from build123d import *

# Parameters (mm, degrees)
F0_R     = 30
F1_DEPTH = 5
F3_DEPTH = 5.001
F4_R     = 9.975
F5_DEPTH = 4.9


with BuildPart() as f1:
    # F0 (on Front) → F1 (new body)
    with BuildSketch(Plane.XZ):
        Circle(F0_R)
    extrude(amount=F1_DEPTH)

    # F2 (on face) → F3 (cut, through all)
    with BuildSketch(Plane.XZ.offset(5)):
        Polygon((-2.601597, 21.949199), (-2.601597, 20.949199), (-2.601597, 19.949199), (2.398403, 19.949199), (2.398403, 21.949199), align=None)
        Polygon((-4.522329, 21.644985), (-9.277612, 20.0999), (-8.968595, 19.148844), (-8.659578, 18.197787), (-3.904295, 19.742872), align=None)
        Polygon((-11.01033, 19.217036), (-15.055415, 16.27811), (-14.467629, 15.469093), (-13.879844, 14.660076), (-9.834759, 17.599002), align=None)
        Polygon((-16.430507, 14.903017), (-19.369434, 10.857932), (-18.560417, 10.270147), (-17.7514, 9.682362), (-14.812473, 13.727447), align=None)
        Polygon((-20.252298, 9.125214), (-21.797383, 4.369932), (-20.846326, 4.060915), (-19.895269, 3.751898), (-18.350185, 8.50718), align=None)
        Polygon((-22.101597, 2.449199), (-22.101597, -2.550801), (-21.101597, -2.550801), (-20.101597, -2.550801), (-20.101597, 2.449199), align=None)
        Polygon((-21.797383, -4.471533), (-20.252298, -9.226816), (-19.301241, -8.917799), (-18.350185, -8.608782), (-19.895269, -3.853499), align=None)
        Polygon((-19.369434, -10.959534), (-16.430507, -15.004619), (-15.62149, -14.416833), (-14.812473, -13.829048), (-17.7514, -9.783963), align=None)
        Polygon((-15.055415, -16.379711), (-11.01033, -19.318638), (-10.422544, -18.509621), (-9.834759, -17.700604), (-13.879844, -14.761677), align=None)
        Polygon((-9.277612, -20.201502), (-4.522329, -21.746587), (-4.213312, -20.79553), (-3.904295, -19.844473), (-8.659578, -18.299389), align=None)
        Polygon((-2.601597, -22.050801), (2.398403, -22.050801), (2.398403, -21.050801), (2.398403, -20.050801), (-2.601597, -20.050801), align=None)
        Polygon((4.319136, -21.746587), (9.074419, -20.201502), (8.765402, -19.250445), (8.456385, -18.299389), (3.701102, -19.844473), align=None)
        Polygon((10.807136, -19.318638), (14.852221, -16.379711), (14.264436, -15.570694), (13.676651, -14.761677), (9.631566, -17.700604), align=None)
        Polygon((16.227314, -15.004619), (19.16624, -10.959534), (18.357223, -10.371748), (17.548206, -9.783963), (14.60928, -13.829048), align=None)
        Polygon((20.049104, -9.226816), (21.594189, -4.471533), (20.643133, -4.162516), (19.692076, -3.853499), (18.146991, -8.608782), align=None)
        Polygon((21.898403, -2.550801), (21.898403, 2.449199), (20.898403, 2.449199), (19.898403, 2.449199), (19.898403, -2.550801), align=None)
        Polygon((21.594189, 4.369932), (20.049104, 9.125214), (19.098048, 8.816197), (18.146991, 8.50718), (19.692076, 3.751898), align=None)
        Polygon((19.16624, 10.857932), (16.227314, 14.903017), (15.418297, 14.315232), (14.60928, 13.727447), (17.548206, 9.682362), align=None)
        Polygon((14.852221, 16.27811), (10.807136, 19.217036), (10.219351, 18.408019), (9.631566, 17.599002), (13.676651, 14.660076), align=None)
        Polygon((9.074419, 20.0999), (4.319136, 21.644985), (4.010119, 20.693929), (3.701102, 19.742872), (8.456385, 18.197787), align=None)
    extrude(amount=-F3_DEPTH, mode=Mode.SUBTRACT)

    # F4 (on face) → F5 (join)
    with BuildSketch(Plane.XZ.offset(5)):
        Circle(F4_R)
    extrude(amount=F5_DEPTH)


solid = f1.part
CAD build for the part. Positions are in the model's coordinates, mm. A direction names the side the tool comes from. Coordinates: 2 decimals unless noted, no trailing zeros. Loops run counter-clockwise (first coordinate to the right, second up) from the corner with the lowest first, then second, coordinate; pieces in that order, holes last. Notation, with made-up numbers: (85, -25) - (97, -25) arc R19 ccw to (97, 5) - close; hole circle Ø3 at (41.5, 26.25). An arc over 180 degrees is marked (long way). Use one line per item in the form item = value. Start each with the question number.
1) Band-saw the part on D-D (x = -12). Give the cut face in (y, z), and give its area (3 significant figures).
2) Flat gauge pins, fed straight in: pin 1 (1.5 mm diameter, centred on x = -0.5, y = -3, fed in from -Z); pin 2 (1.5 mm diameter, centred on x = -1, y = -2, fed in from +Z); pin 3 (1.6 mm diameter, centred on x = 21, y = -2, fed in from +Z). Where does each tip first touch, or does it go through?
3) Band-saw the part on C-C (y = -1). State how many separate pieces and enclosed holes the cut face has, and give its area (3 significant figures).
4) Band-saw the part on B-B (x = 0). Give the cut face in (y, z) (3 decimals), and give its area (3 significant figures).
5) Two-plate mould, pull along X, no slides. Class faces 1 (the face through (13, -5, 0)), 2 (the face through (-20.86, -2.535, 4.065)): +X half, -X half, draft (parallel to the pull), parting line (faces both ways), or undercut.
6) Drill centre lines: L1, parallel to Z at x = -8, y = -1.25; L2, parallel to X at y = -3, z = 6; L3, parallel to X at y = -2.75, z = 10.5. Where is each one in solid material? Low to high. Write a range as from..to.
7) Tool access for faces 3 (the face through (0, -9.9, 0)), 4 (the face through (6.11, -2.54, -19.06)): list every direction of +Z, -Z, +X, -X, +Y, -Y with a clear straight run to the whole face (end or side of a thin tool).
8) Band-saw the part on A-A (z = 0). Give the cut face in (x, y) (3 decimals), and give its area (3 significant figures).
Check values:
q1.outline = (-5, -27.5) - (0, -27.5) - (0, -18.6) - (-5, -18.6) - close; (-5, -16.13) - (0, -16.13) - (0, 16.03) - (-5, 16.03) - close; (-5, 18.5) - (0, 18.5) - (0, 27.5) - (-5, 27.5) - close
q1.area = 250 mm2
q2.pin_1 = -30
q2.pin_2 = 30
q2.pin_3 = 22.18
q3.separate_pieces = 1
q3.enclosed_holes = 20
q3.area = 2,630 mm2
q4.outline = (-9.9, -9.975) - (-5, -9.975) - (-5, -20.051) - (0, -20.051) - (0, 19.949) - (-5, 19.949) - (-5, 9.975) - (-9.9, 9.975) - close; (-5, -30) - (0, -30) - (0, -22.051) - (-5, -22.051) - close; (-5, 21.949) - (0, 21.949) - (0, 30) - (-5, 30) - close
q4.area = 378 mm2
q5.face_1 = draft
q5.face_2 = undercut
q6.L1 = -28.91..-20.62, -18.51..18.41, 20.52..28.91
q6.L2 = -29.39..-21.27, -19.16..18.96, 21.06..29.39
q6.L3 = -28.1..-18.88, -17.16..16.95, 18.67..28.1
q7.face_3 = +Z, -Z, +X, -X, -Y
q7.face_4 = +Y, -Y
q8.outline = (-30, -5) - (-22.102, -5) - (-22.102, 0) - (-30, 0) - close; (-20.102, -5) - (-9.975, -5) - (-9.975, -9.9) - (9.975, -9.9) - (9.975, -5) - (19.898, -5) - (19.898, 0) - (-20.102, 0) - close; (21.898, -5) - (30, -5) - (30, 0) - (21.898, 0) - close
q8.area = 378 mm2
